```python
from build123d import *

# Parameters (mm, degrees)
SKETCH1_W           = 38
SKETCH1_H           = 38
BOSS_EXTRUDE1_DEPTH = 3
SKETCH2_W           = 38
SKETCH2_H           = 38
BOSS_EXTRUDE2_DEPTH = 4


with BuildPart() as part:
    # Sketch1 → Boss-Extrude1 (new body)
    with BuildSketch(Plane(origin=(0, 0, 0), x_dir=(1, 0, 0), z_dir=(0, 1, 0))):
        with Locations((19, 19)):
            Rectangle(SKETCH1_W, SKETCH1_H)
        with BuildLine():
            Line((14, 34), (24, 34))
            ThreePointArc((24, 34), (31.071067812, 31.071067812), (34, 24))
            Line((34, 24), (34, 14))
            ThreePointArc((34, 14), (31.071067812, 6.928932188), (24, 4))
            Line((24, 4), (14, 4))
            ThreePointArc((14, 4), (6.928932188, 6.928932188), (4, 14))
            Line((4, 14), (4, 24))
            ThreePointArc((4, 24), (6.928932188, 31.071067812), (14, 34))
        make_face(mode=Mode.SUBTRACT)
    extrude(amount=BOSS_EXTRUDE1_DEPTH)

    # Sketch2 → Boss-Extrude2 (add)
    with BuildSketch(Plane(origin=(0, 3, 0), x_dir=(1, 0, 0), z_dir=(0, 1, 0))):
        with Locations((19, 19)):
            Rectangle(SKETCH2_W, SKETCH2_H)
        with BuildLine():
            Line((12, 36), (26, 36))
            ThreePointArc((26, 36), (33.071067812, 33.071067812), (36, 26))
            Line((36, 26), (36, 12))
            ThreePointArc((36, 12), (33.071067812, 4.928932188), (26, 2))
            Line((26, 2), (12, 2))
            ThreePointArc((12, 2), (4.928932188, 4.928932188), (2, 12))
            Line((2, 12), (2, 26))
            ThreePointArc((2, 26), (4.928932188, 33.071067812), (12, 36))
        make_face(mode=Mode.SUBTRACT)
    extrude(amount=BOSS_EXTRUDE2_DEPTH)


solid = part.part
```
For this review, take the finished solid that the model builds, in its own axes (mm). A direction names the side the tool comes from. Give positions to 0.01 mm unless a question says otherwise; leave off trailing zeros. Write each loop counter-clockwise with the first axis right and the second up, starting at its lowest first coordinate (ties: lowest second). Pieces come first, ordered by that corner, then holes. Notation, with made-up numbers: M 18.5,-1.75 L 38.5,-1.75 A16 ccw 38.5,19.25 Z; hole C 69,73.25 d2. An arc over 180 degrees is marked long. One line per item, written item: value.
1) Take a section at A-A, the plane z = -22. Write out the cut boundary in (x, y), then the cut area to 3 significant figures.
Results are:
outline: M 0,0 L 4,0 L 4,3 L 2,3 L 2,7 L 0,7 Z; M 34,0 L 38,0 L 38,7 L 36,7 L 36,3 L 34,3 Z
area: 40.0 mm²
2) Take a section at B-B, the plane x = 16.5. Write out the cut boundary in (y, z).
Results are:
outline: M 0,-38 L 7,-38 L 7,-36 L 3,-36 L 3,-34 L 0,-34 Z; M 0,-4 L 3,-4 L 3,-2 L 7,-2 L 7,0 L 0,0 Z
3) The part is to be moulded in two halves that separate along X. For faces 1 (the flat face through (2, 0, -19)), 2 (the flat face through (19, 5, -2)), 3 (the flat face through (0, 3, -19)), say which applies: +X half, -X half, draft (parallel to the pull), parting line (faces both ways), or undercut.
Results are:
face 1: draft
face 2: undercut
face 3: -X half
4) For faces 4 (the flat face through (19, 7, -37)), 5 (the flat face through (19, 1, -34)), 6 (the flat face through (18.9, 3, -34.2)), list the 3-axis set-ups (+Z, -Z, +X, -X, +Y, -Y) from which the entire face can be reached by the end or side of a thin tool; tool diameter is ignored.
Results are:
face 4: +Z, -Z, +X, -X, +Y
face 5: +Y, -Y
face 6: +Y
5) Take a section at C-C, the plane y = 6. Write out the cut boundary in (x, z), then the cut area to 3 significant figures.
Results are:
outline: M 0,-38 L 38,-38 L 38,0 L 0,0 Z; hole M 2,-26 A10 ccw 12,-36 L 26,-36 A10 ccw 36,-26 L 36,-12 A10 ccw 26,-2 L 12,-2 A10 ccw 2,-12 Z
area: 374 mm²
6) For line 1 (X direction, y = 3.5, z = -21.5); line 2 (Z direction, x = 14.5, y = 1); line 3 (Z direction, x = 14, y = 4), list the stretches that pass through material, from the lowest coordinate up. Write a range as from..to.
Results are:
line 1: x = 0..2, 36..38
line 2: z = -38..-34, -4..0
line 3: z = -38..-36, -2..0
7) Take a section at D-D, the plane y = 2. Write out the cut boundary in (x, z).
Results are:
outline: M 0,-38 L 38,-38 L 38,0 L 0,0 Z; hole M 4,-24 A10 ccw 14,-34 L 24,-34 A10 ccw 34,-24 L 34,-14 A10 ccw 24,-4 L 14,-4 A10 ccw 4,-14 Z
